Geometry check sheet. Reference: the model listing, model coordinates, mm. Give positions to 0.01 mm unless a question says otherwise; leave off trailing zeros. Answer as CSV lines item,"result".
from build123d import *

# Parameters (mm, degrees)
PAD_DEPTH    = 730
SKETCH001_R  = 12.5
POCKET_DEPTH = 15


with BuildPart() as part:
    # Sketch → Pad (new body)
    with BuildSketch(Plane.YZ):
        with BuildLine():
            Line((-209.5, 0), (209.5, 0))
            Line((209.5, 0), (209.5, 220))
            ThreePointArc((209.5, 220), (206.571068, 227.071068), (199.5, 230))
            Line((199.5, 230), (-199.5, 230))
            ThreePointArc((-199.5, 230), (-206.571068, 227.071068), (-209.5, 220))
            Line((-209.5, 220), (-209.5, 0))
        make_face()
    extrude(amount=PAD_DEPTH)

    # Sketch001 → Pocket (cut)
    with BuildSketch(Plane.YZ):
        with Locations((139.5, 70)):
            Circle(SKETCH001_R)
    extrude(amount=POCKET_DEPTH, mode=Mode.SUBTRACT)


solid = part.part
(1) Draft check along Y on faces 1 (the face through (7.395, 151.423, 73.755)), 2 (the face through (15, 139, 70)), 3 (the face through (360, -209.5, 112)), 4 (the face through (360, 3, 230)). Enter one of: +Y half, -Y half, draft (parallel to the pull), parting line (faces both ways), or undercut.
The answers:
face 1,"undercut"
face 2,"undercut"
face 3,"-Y half"
face 4,"draft"
(2) Gauge pin test, flat end, axial feed: P1, Ø12.5, axis at y = 144.5, z = 70, coming from the -X side. Record the tip position at first contact, or that the pin passes through.
The answers:
P1,"stops at x = 15"
(3) Material ranges on line 1 (Z direction, x = 8.75, y = 139.5), recorded low to high.
The answers:
line 1,"z = 0 to 57.5, 82.5 to 230"
